For this review, take the finished solid that the model builds, in its own axes (mm). A direction names the side the tool comes from. Give positions to 0.01 mm unless a question says otherwise; leave off trailing zeros. Loops run counter-clockwise (first coordinate to the right, second up) from the corner with the lowest first, then second, coordinate; pieces in that order, holes last. Notation, with made-up numbers: M 71.5,63 L 77.5,63 A20 ccw 77.5,85 Z; hole C 43,59.25 d11. An arc over 180 degrees is marked long. Use CSV: the item, a comma, the result in double quotes. Start each with the question number.
1. Tool access review of faces 5 (the face through (-390, 2, 100)), 6 (the face through (-53, -25.357, 227)), 7 (the face through (-46.9, 0, 225.7)), 8 (the face through (-50, 24.643, 227)): name each direction out of +Z, -Z, +X, -X, +Y, -Y from which nothing blocks a thin tool from reaching the whole face with its end or side.
2. Insertion check: P1, Ø15, axis at y = 2, z = 149, coming from the +X side; P2, Ø6, axis at x = -254.5, z = 196, coming from the +Y side; P3, Ø12, axis at x = -61.5, y = -30.5, coming from the +Z side. Each pin has a flat end and moves straight along its axis. Give the tip position at first contact, or say it passes through.
3. Take a section at C-C, the plane x = 425. Write out the cut boundary in (y, z).
4. Take a section at B-B, the plane y = 11. Write out the cut boundary in (x, z), and give its area (3 significant figures).
5. The part is to be moulded in two halves that separate along X. For faces 1 (the face through (453.615, 7.741, 287.675)), 2 (the face through (453.615, 7.741, 12.675)), 3 (the face through (-78.46, -0.01, 249.3)), 4 (the face through (-255.951, 0, 150)), say which applies: pulls with the +X half, pulls with the -X half, needs draft (parallel to the pull), parting line crosses it, or undercut.
6. To check wall thickness, follow line 1 (Y direction, x = 425, z = 15.25); line 2 (Z direction, x = 259, y = 4.5); line 3 (Y direction, x = -292, z = 176.5). State the ranges of each line that lie inside material, in increasing order. Write a range as [from, to].
7. Take a section at D-D, the plane x = -234. Write out the cut boundary in (y, z).
8. Take a section at A-A, the plane x = 230.5. Write out the cut boundary in (y, z).
from build123d import *

# Parameters (mm, degrees)
BOSS_EXTRUDE1_DEPTH = 300
SKETCH3_OUTSIDE_W   = 1151.978
SKETCH3_OUTSIDE_H   = 502.25
CUT_EXTRUDE1_DEPTH  = 300
CUT_EXTRUDE3_DEPTH  = 300
SKETCH6_R           = 30
CUT_EXTRUDE4_DEPTH  = 200


with BuildPart() as part:
    # Sketch1 → Boss-Extrude1 (new body)
    with BuildSketch(Plane.XY):
        with BuildLine():
            Line((350.126678984, 24.643496119), (-349.873321016, 24.643496119))
            Line((-349.873321016, 24.643496119), (-405.7801007, 47.538028277))
            ThreePointArc((-405.7801007, 47.538028277), (-474.713018176, 2.509970806), (-408.102340797, -45.887247404))
            Line((-408.102340797, -45.887247404), (-349.873321016, -25.356503881))
            Line((-349.873321016, -25.356503881), (350.126678984, -25.356503881))
            Line((350.126678984, -25.356503881), (406.56125394, -47.746215249))
            ThreePointArc((406.56125394, -47.746215249), (474.7986376, -5.753101083), (415.157857426, 47.751473547))
            Line((415.157857426, 47.751473547), (401.702587644, 42.970319678))
            Line((401.702587644, 42.970319678), (350.126678984, 24.643496119))
        make_face()
    extrude(amount=BOSS_EXTRUDE1_DEPTH)

    # Sketch3 outside → Cut-Extrude1 (cut)
    with BuildSketch(Plane(origin=(0, 24.643496119, 0), x_dir=(1, 0, 0), z_dir=(0, 1, 0))):
        with Locations((0.136, -150)):
            Rectangle(SKETCH3_OUTSIDE_W, SKETCH3_OUTSIDE_H)
        Polygon((156.384680345, -275), (-255.951397242, -175), (-255.951397242, -150), (-255.951397242, -125), (156.384680345, -25), (646.790959518, -25), (660.003845731, 0), (156.384680345, 0), (-306.817002614, -100), (-623.605485165, -100), (-623.605485165, -200), (-306.817002614, -200), (156.384680345, -300), (568.093933709, -300), (523.266387174, -275), align=None, mode=Mode.SUBTRACT)
    extrude(amount=-CUT_EXTRUDE1_DEPTH, mode=Mode.SUBTRACT)

    # Sketch5 → Cut-Extrude3 (cut)
    with BuildSketch(Plane(origin=(0, 24.643496119, 0), x_dir=(1, 0, 0), z_dir=(0, 1, 0))):
        Polygon((156.384680345, -25), (555.921134312, -25), (555.921134312, -275), (156.384680345, -275), (-255.951397242, -175), (-255.951397242, -125), align=None)
        Polygon((-349.873321016, -100), (-477.733615617, -100), (-477.733615617, 50.340527991), (-332.07706739, 50.340527991), align=None)
        Polygon((-349.873321016, -200), (-349.873321016, -364.123748435), (-511.890412396, -324.647411731), (-481.519399358, -200), align=None)
    extrude(amount=CUT_EXTRUDE3_DEPTH, mode=Mode.SUBTRACT)

    # Sketch6 → Cut-Extrude4 (cut, symmetric)
    with BuildSketch(Plane.XY.offset(200)):
        with Locations((-424.728457358, 1.267521688)):
            Circle(SKETCH6_R)
        with Locations((425, -1.27027907)):
            Circle(SKETCH6_R)
    extrude(amount=CUT_EXTRUDE4_DEPTH, both=True, mode=Mode.SUBTRACT)


solid = part.part
Result set:
1,face 5,"-Z, -X, +Y, -Y"
1,face 6,"+Z, -Z, -Y"
1,face 7,"+X, +Y, -Y"
1,face 8,"+Z, -Z, +Y"
2,P1,"x = -255.95"
2,P2,"y = 24.64"
2,P3,"z = 253.63"
3,outline,"M -51.27,0 L -31.27,0 L -31.27,25 L -51.27,25 Z; M -51.27,275 L -31.27,275 L -31.27,300 L -51.27,300 Z; M 28.73,0 L 48.73,0 L 48.73,25 L 28.73,25 Z; M 28.73,275 L 48.73,275 L 48.73,300 L 28.73,300 Z"
4,outline,"M -473.77,100 L -453.11,100 L -453.11,200 L -473.77,200 Z; M -396.35,100 L -306.82,100 L 156.38,0 L 397.62,0 L 397.62,25 L 156.38,25 L -255.95,125 L -255.95,175 L 156.38,275 L 397.62,275 L 397.62,300 L 156.38,300 L -306.82,200 L -396.35,200 Z; M 452.38,0 L 473.47,0 L 473.47,25 L 452.38,25 Z; M 452.38,275 L 473.47,275 L 473.47,300 L 452.38,300 Z"
4,area,"54,900 mm2"
5,face 1,"undercut"
5,face 2,"undercut"
5,face 3,"pulls with the -X half"
5,face 4,"pulls with the +X half"
6,line 1,"[-51.27, -31.27], [28.73, 48.73]"
6,line 2,"[0, 25], [275, 300]"
6,line 3,"[-25.36, 24.64]"
7,outline,"M -25.36,84.28 L 24.64,84.28 L 24.64,119.68 L -25.36,119.68 Z; M -25.36,180.32 L 24.64,180.32 L 24.64,215.72 L -25.36,215.72 Z"
8,outline,"M -25.36,0 L 24.64,0 L 24.64,25 L -25.36,25 Z; M -25.36,275 L 24.64,275 L 24.64,300 L -25.36,300 Z"
